Autodesk Inventor part; units mm, degrees
ref_plane "YZ Plane" through (0, 0, 0) normal (1, 0, 0) x (0, 1, 0)
ref_plane "XZ Plane" through (0, 0, 0) normal (0, 1, 0) x (-1, 0, 0)
ref_plane "XY Plane" through (0, 0, 0) normal (0, 0, 1) x (1, 0, 0)
sketch "Boceto1" plane through (0, 0, 0) normal (0, 0, 1) x (1, 0, 0)
  line L0 (0, 0) -> (40, 0)
  line L1 (40, 0) -> (40, -40)
  line L2 (40, -40) -> (0, -40)
  line L3 (0, -40) -> (0, 0)
  dimension "d0" = 40
  dimension "d1" = 40
extrude "Extrusión1" add sketch "Boceto1" along normal blind 120
sketch "Boceto2" plane through (0, 0, 120) normal (0, 0, 1) x (1, 0, 0)
  circle A0 centre (20, -20) radius 10
  line L0 (0, 0) -> (0, -40)
  line L1 (40, 0) -> (0, 0)
  dimension "d4" = 20
  dimension "d5" = 20
  dimension "d6" = 20
extrude "Extrusión2" cut sketch "Boceto2" against normal blind 100
ref_plane "Plano de trabajo1" through (20, -40, 0) normal (-1, 0, 0) x (0, 0, 1)
sketch "Boceto5" plane through (20, -40, 0) normal (-1, 0, 0) x (0, 0, 1)
  line L0 (0, 0) -> (0, 40)
  line L1 (0, 30) -> (-15, 30)
  line L2 (-15, 30) -> (-15, 10)
  line L3 (-15, 10) -> (0, 10)
  line L4 (0, 10) -> (0, 30)
  line L5 (0, 40) -> (120, 40)
  circle A0 centre (-15, 20) radius 10
  dimension "d10" = 15
  dimension "d11" = 20
  dimension "d12" = 30
extrude "Extrusión3" add sketch "Boceto5" along normal mid plane 12
hole "Agujero1" at (14, -19.1963, -18.9315) direction (1, 0, 0) diameter 8 end through all
properties part number "cilindro sierra"
Part model, mm, in its own coordinate system. A direction names the side the tool comes from. Coordinates: 2 decimals unless noted, no trailing zeros. Write each loop counter-clockwise with the first axis right and the second up, starting at its lowest first coordinate (ties: lowest second). Pieces come first, ordered by that corner, then holes. Notation, with made-up numbers: (84, 76) - (99, 76) arc R17 cw to (99, 93) - close; hole circle Ø8 at (9, 25.25). An arc over 180 degrees is marked (long way). Put each result on its own line as item: value.
1. Band-saw the part on A-A (y = -17.5). Write the cut outline in (x, z).
Final values:
outline: (0, 0) - (14, 0) - (14, -15.31) - (26, -15.31) - (26, 0) - (40, 0) - (40, 120) - (29.68, 120) - (29.68, 20) - (10.32, 20) - (10.32, 120) - (0, 120) - close; (14, -24.68) - (26, -24.68) - (26, -22.55) - (14, -22.55) - close
2. 3-axis set-ups, long thin cutter, end or side, ignore diameter. For faces 4 (the flat face through (20, -20, 20)), 5 (the flat face through (20, -10, -7)), 6 (the flat face through (14, -20, -10)), 7 (the flat face through (20, -30, -8)): which of +Z, -Z, +X, -X, +Y, -Y reach the whole face in a straight line?
Final values:
face 4: +Z
face 5: -Z, +X, -X, +Y
face 6: -Z, -X, +Y, -Y
face 7: -Z, +X, -X, -Y
3. Flat gauge pins, fed straight in: pin 1 Ø3 at (x, z) = (10, 57) entering from +Y; pin 2 Ø10.5 at (y, z) = (-19.2, -18.93) entering from -X; pin 3 Ø6 at (y, z) = (-17, -13.5) entering from +X; pin 4 Ø9.5 at (x, z) = (18.5, -8) entering from +Y. Where does each tip first touch, or does it go through?
Final values:
pin 1: stops at y = 0
pin 2: stops at x = 14
pin 3: stops at x = 26
pin 4: stops at y = -10
4. Probe line 1 along Y through (x, z) = (20, 42); line 2 along Z through (x, y) = (21.5, -19.5); line 3 along X through (y, z) = (-20.5, 39). List the from-to ranges inside material, lowest first. Write a range as [from, to].
Final values:
line 1: y = [-40, -30], [-10, 0]
line 2: z = [-24.99, -22.92], [-14.94, 20]
line 3: x = [0, 10.01], [29.99, 40]
5. Band-saw the part on C-C (x = 20). Write the cut outline in (y, z).
Final values:
outline: (-40, 0) - (-30, 0) - (-30, -15) arc R10 ccw to (-10, -15) - (-10, 0) - (0, 0) - (0, 120) - (-10, 120) - (-10, 20) - (-30, 20) - (-30, 120) - (-40, 120) - close; hole circle Ø8 at (-19.2, -18.93)
6. Band-saw the part on D-D (y = -27.5). Write the cut outline in (x, z).
Final values:
outline: (0, 0) - (14, 0) - (14, -21.61) - (26, -21.61) - (26, 0) - (40, 0) - (40, 120) - (26.61, 120) - (26.61, 20) - (13.39, 20) - (13.39, 120) - (0, 120) - close
7. Two-plate mould, pull along Z, no slides. Class faces 1 (the flat face through (26, -20, -10)), 2 (the cylindrical face through (20.084, -23.162, -19.452)), 3 (the cylindrical face through (20, -20, -25)): +Z half, -Z half, draft (parallel to the pull), parting line (faces both ways), or undercut.
Final values:
face 1: draft
face 2: undercut
face 3: -Z half
8. Band-saw the part on B-B (z = 45). Write the cut outline in (x, y), then the cut area to 3 significant figures.
Final values:
outline: (0, -40) - (40, -40) - (40, 0) - (0, 0) - close; hole circle Ø20 at (20, -20)
area: 1,290 mm²
